The model under review builds one solid part; all positions refer to its coordinate system, in mm. A direction names the side the tool comes from. Coordinates: 2 decimals unless noted, no trailing zeros. Loops run counter-clockwise (first coordinate to the right, second up) from the corner with the lowest first, then second, coordinate; pieces in that order, holes last. Notation, with made-up numbers: M 3.5,-15.5 L 29.5,-15.5 A30 ccw 29.5,7.5 Z; hole C -31,-10.5 d5. An arc over 180 degrees is marked long. Use one line per item in the form item = value.
```python
from build123d import *

# Parameters (mm, degrees)
F1_DEPTH = 88.9
F2_R     = 5.08
F4_DEPTH = 103.378


with BuildPart() as f1:
    # F0 (on Front) → F1 (new body)
    with BuildSketch(Plane.XZ):
        Polygon((6.59128, 64.89383), (6.59128, 68.06883), (-18.80872, 68.06883), (-18.80872, -12.32217), (6.59128, -12.32217), (6.59128, -9.14717), (-15.63372, -9.14717), (-15.63372, 64.89383), align=None)
    extrude(amount=F1_DEPTH)

    # F2
    f2_edges = [f1.edges().sort_by_distance(p)[0] for p in [
        (-18.80872, -44.45, 68.06883),
        (-18.80872, -44.45, -12.32217),
    ]]
    fillet(f2_edges, radius=F2_R)

    # F3 (on face) → F4 (cut)
    with BuildSketch(Plane.XY.offset(68.06883)):
        Polygon((6.59128, 0), (-13.72872, 0), (6.59128, -11.731757), align=None)
    extrude(amount=-F4_DEPTH, mode=Mode.SUBTRACT)


solid = f1.part
```
1. Wall thickness on line 1 along Z through (x, y) = (-9, -63); line 2 along X through (y, z) = (-73.5, 31); line 3 along Z through (x, y) = (-17, -23.5): over which ranges is each line inside the solid? List them lowest first. Write a range as from..to.
Response values:
line_1 = -12.32..-9.15, 64.89..68.07
line_2 = -18.81..-15.63
line_3 = -11.13..66.88
2. Machinability: for faces 1 (the face through (-4, -44, -9.147)), 2 (the face through (-17.3, -45.1, 66.6)), which of the approach directions +Z, -Z, +X, -X, +Y, -Y give a long, thin tool a straight path to every point of the face, cutting with its end or side? Answer none if there is none.
Response values:
face_1 = +X, +Y, -Y
face_2 = +Z, -X, +Y, -Y
3. Add section A-A (y = -56.5). State the section outline as (x, z) points, then the cut area to 3 significant figures.
Response values:
outline = M -18.81,-7.24 A5.08 ccw -13.73,-12.32 L 6.59,-12.32 L 6.59,-9.15 L -15.63,-9.15 L -15.63,64.89 L 6.59,64.89 L 6.59,68.07 L -13.73,68.07 A5.08 ccw -18.81,62.99 Z
area = 385 mm^2
4. Insertion check: P1, Ø1, axis at y = -27.5, z = 13.5, coming from the +X side; P2, Ø8, axis at x = -13.5, z = -0.5, coming from the +Y side. Each pin has a flat end and moves straight along its axis. Give the tip position at first contact, or say it passes through.
Response values:
P1 = -15.63
P2 = 0
5. The part is to be moulded in two halves that separate along Z. For faces 3 (the face through (-5, -44, 64.894)), 4 (the face through (-17.36, -45.072, -10.795)), 5 (the face through (-18.809, -44, 28)), say which applies: pulls with the +Z half, pulls with the -Z half, needs draft (parallel to the pull), parting line crosses it, or undercut.
Response values:
face_3 = undercut
face_4 = pulls with the -Z half
face_5 = needs draft
6. Add section C-C (z = 14.5). State the section outline as (x, y) points, then the cut area to 3 significant figures.
Response values:
outline = M -18.81,-88.9 L -15.63,-88.9 L -15.63,0 L -18.81,0 Z
area = 282 mm^2
7. Add section B-B (x = -6.5). State the section outline as (y, z) points.
Response values:
outline = M -88.9,-12.32 L -4.17,-12.32 L -4.17,-9.15 L -88.9,-9.15 Z; M -88.9,64.89 L -4.17,64.89 L -4.17,68.07 L -88.9,68.07 Z
